from build123d import *

# Parameters (mm, degrees)
SKETCH1_R           = 7.75
SKETCH1_R_2         = 3.875
BOSS_EXTRUDE1_DEPTH = 1
SKETCH2_R           = 6.75
SKETCH2_R_2         = 3.875
BOSS_EXTRUDE2_DEPTH = 3.5
CHAMFER1_SIZE       = 1


with BuildPart() as part:
    # Sketch1 → Boss-Extrude1 (new body)
    with BuildSketch(Plane.XY):
        Circle(SKETCH1_R)
        Circle(SKETCH1_R_2, mode=Mode.SUBTRACT)
    extrude(amount=BOSS_EXTRUDE1_DEPTH)

    # Sketch2 → Boss-Extrude2 (add)
    with BuildSketch(Plane.XY.offset(1)):
        Circle(SKETCH2_R)
        Circle(SKETCH2_R_2, mode=Mode.SUBTRACT)
    extrude(amount=BOSS_EXTRUDE2_DEPTH)

    # Chamfer1
    chamfer1_edges = [part.edges().sort_by_distance(p)[0] for p in [
        (-6.75, 0, 1),
    ]]
    chamfer(chamfer1_edges, length=CHAMFER1_SIZE - 0.0001)  # a hair under: the kernel refuses the full size

    # Mirror5: part across plane


with BuildPart() as part_1:
    add(part.part)
    add(part.part.mirror(Plane.XY.offset(4.5)))


solid = part_1.part
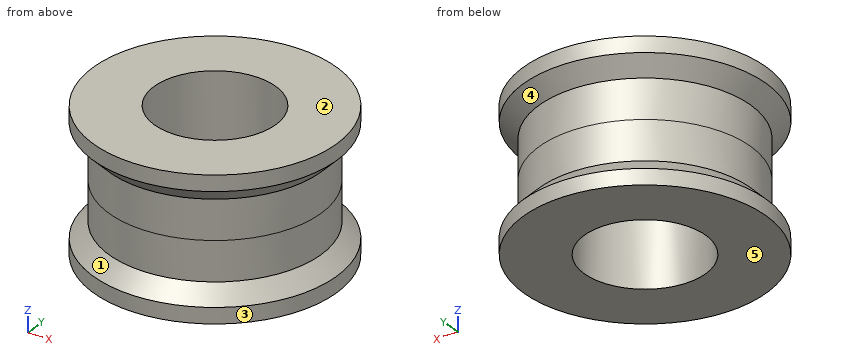
Geometry check sheet. Reference: the model listing, model coordinates, mm. Face numbers are marked on the shaded views. A direction names the side the tool comes from. Round coordinates to 2 decimals unless told otherwise and drop trailing zeros. Order: outer loops, then holes, each group sorted by start corner. A loop starts at its lowest first (then second) coordinate and runs counter-clockwise, first axis right, second up. Notation, with made-up numbers: (15.25, -24.5) -> (69.25, -24.5) arc R28 cw to (69.25, -2.5) -> close; hole circle Ø7 at (15, 76.25). An arc over 180 degrees is marked (long way). Use one line per item in the form item = value.
1. Set-up check for the marked faces 4 and 5: record each of +Z, -Z, +X, -X, +Y, -Y from which the full face is reachable in a straight line by a thin tool's end or side.
Working result:
face_4 = none
face_5 = -Z, +X, -X, +Y, -Y
2. Mould release check, pull along Z, two halves, no side actions. Record for the marked faces 1, 2 and 3: pulls with the +Z half, pulls with the -Z half, needs draft (parallel to the pull), parting line crosses it, or undercut.
Working result:
face_1 = undercut
face_2 = pulls with the +Z half
face_3 = needs draft
3. Scan lines: line 1 along Y through (x, z) = (0, 2.9) (3 decimals); line 2 along X through (y, z) = (2.5, 6.75); line 3 along Y through (x, z) = (-0.5, 6). Record each from-to range of solid material in increasing order. Write a range as from..to.
Working result:
line_1 = -6.75..-3.875, 3.875..6.75
line_2 = -6.27..-2.96, 2.96..6.27
line_3 = -6.73..-3.84, 3.84..6.73
4. Cross-section at D-D, the plane z = 5.25. Enter the section's corners in (x, y) (3 decimals), plus the area to 3 significant figures.
Working result:
outline = circle Ø13.5 at (0, 0); hole circle Ø7.75 at (0, 0)
area = 96.0 mm^2
5. Go/stop test with flat-tipped pins: pin 1 (2 mm diameter, centred on x = 2, z = 2, fed in from +Y); pin 2 (5 mm diameter, centred on y = -5.5, z = 1, fed in from +X). Record where each tip stops, or that it passes through.
Working result:
pin_1 = 7.52
pin_2 = 7.15
6. Cross-section at C-C, the plane z = 8.25. Enter the section's corners in (x, y) (3 decimals).
Working result:
outline = circle Ø15.5 at (0, 0); hole circle Ø7.75 at (0, 0)
